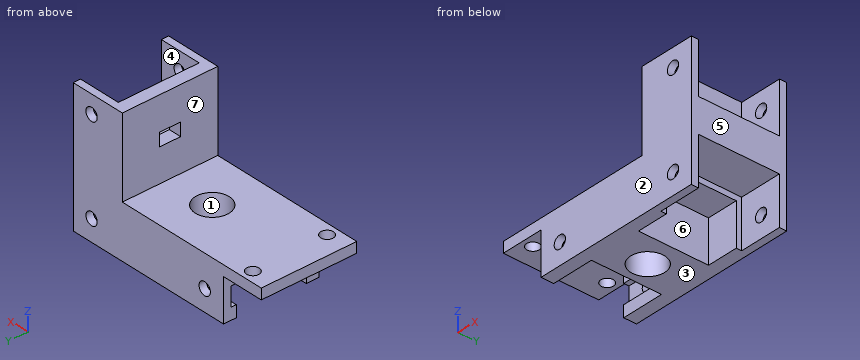
```python
from build123d import *

# Parameters (mm, degrees)
SKETCH1_W               = 36.85
SKETCH1_H               = 22.5
BOSS_EXTRUDE1_DEPTH     = 2.5
SKETCH2_W               = 21.3
SKETCH2_H               = 22.5
BOSS_EXTRUDE2_DEPTH     = 3
SKETCH3_W               = 21.3
SKETCH3_H               = 3
BOSS_EXTRUDE3_DEPTH     = 10
SKETCH4_W               = 49.85
SKETCH4_H               = 3
BOSS_EXTRUDE4_DEPTH     = 10
SKETCH8_W               = 3.1
SKETCH8_H               = 5
CUT_EXTRUDE1_DEPTH      = 5
SKETCH9_R               = 4
SKETCH9_R_2             = 1.5
CUT_EXTRUDE2_DEPTH      = 25
SKETCH11_W              = 10
SKETCH11_H              = 3
CUT_EXTRUDE3_DEPTH      = 10
SKETCH12_R              = 1.5
CUT_EXTRUDE4_DEPTH      = 10
SKETCH14_W              = 12.5
SKETCH14_H              = 10
SKETCH14_W_2            = 10
SKETCH14_H_2            = 8
BOSS_EXTRUDE8_DEPTH     = 19.5
SKETCH13_R              = 1.5
BOSS_EXTRUDE7_DEPTH     = 3
SKETCH15_R              = 4
CUT_EXTRUDE5_DEPTH      = 43
CUT_EXTRUDE6_DEPTH      = 17.7525
CUT_EXTRUDE6_DEPTH_BACK = 1.25
SKETCH16_W              = 10
SKETCH16_H              = 4.5
SKETCH17_W              = 14.131300264
SKETCH17_H              = 19.05
SKETCH17_W_2            = 13.234553728
CUT_EXTRUDE7_DEPTH      = 10


with BuildPart() as part:
    # Sketch1 → Boss-Extrude1 (new body)
    with BuildSketch(Plane.XY):
        with Locations((18.425, 11.25)):
            Rectangle(SKETCH1_W, SKETCH1_H)
    extrude(amount=BOSS_EXTRUDE1_DEPTH)

    # Sketch2 → Boss-Extrude2 (add)
    with BuildSketch(Plane(origin=(36.85, 0, 0), x_dir=(0, 0, -1), z_dir=(1, 0, 0))):
        with Locations((-10.65, 11.25)):
            Rectangle(SKETCH2_W, SKETCH2_H)
    extrude(amount=BOSS_EXTRUDE2_DEPTH)

    # Sketch3 → Boss-Extrude3 (add)
    with BuildSketch(Plane(origin=(39.85, 0, 0), x_dir=(0, 0, -1), z_dir=(1, 0, 0))):
        with Locations((-10.65, 1.5)):
            Rectangle(SKETCH3_W, SKETCH3_H)
    extrude(amount=BOSS_EXTRUDE3_DEPTH)

    # Sketch4 → Boss-Extrude4 (add)
    with BuildSketch(Plane(origin=(0, 0, 0), x_dir=(-1, 0, 0), z_dir=(0, 0, -1))):
        with Locations((-24.925, 1.5)):
            Rectangle(SKETCH4_W, SKETCH4_H)
    extrude(amount=BOSS_EXTRUDE4_DEPTH)

    # Sketch8 → Cut-Extrude1 (cut)
    with BuildSketch(Plane(origin=(39.85, 0, 0), x_dir=(0, 0, -1), z_dir=(1, 0, 0))):
        with Locations((-11.85, 11.25)):
            Rectangle(SKETCH8_W, SKETCH8_H)
    extrude(amount=-CUT_EXTRUDE1_DEPTH, mode=Mode.SUBTRACT)

    # Sketch9 → Cut-Extrude2 (cut)
    with BuildSketch(Plane.XY.offset(2.5)):
        with Locations((25.65, 11.25)):
            Circle(SKETCH9_R)
        with Locations((5.05, 20)):
            Circle(SKETCH9_R_2)
        with Locations((5.05, 2.5)):
            Circle(SKETCH9_R_2)
    extrude(amount=-CUT_EXTRUDE2_DEPTH, mode=Mode.SUBTRACT)

    # Sketch11 → Cut-Extrude3 (cut)
    with BuildSketch(Plane(origin=(0, 0, -10), x_dir=(-1, 0, 0), z_dir=(0, 0, -1))):
        with Locations((-5, 1.5)):
            Rectangle(SKETCH11_W, SKETCH11_H)
    extrude(amount=-CUT_EXTRUDE3_DEPTH, mode=Mode.SUBTRACT)

    # Sketch12 → Cut-Extrude4 (cut)
    with BuildSketch(Plane(origin=(0, 3, 0), x_dir=(1, 0, 0), z_dir=(0, 1, 0))):
        with Locations(Location((15, 5, 0), (0, 0, 270))):
            Circle(SKETCH12_R)
        with Locations(Location((45, 5, 0), (0, 0, 270))):
            Circle(SKETCH12_R)
        with Locations(Location((45, -17, 0), (0, 0, 270))):
            Circle(SKETCH12_R)
    extrude(amount=-CUT_EXTRUDE4_DEPTH, mode=Mode.SUBTRACT)

    # Sketch14 → Boss-Extrude8 (add)
    with BuildSketch(Plane(origin=(0, 3, 0), x_dir=(1, 0, 0), z_dir=(0, 1, 0))):
        with Locations((26.25, 5)):
            Rectangle(SKETCH14_W, SKETCH14_H)
        with Locations((44.85, -5.3)):
            Rectangle(SKETCH14_W_2, SKETCH14_H_2)
    extrude(amount=BOSS_EXTRUDE8_DEPTH)

    # Sketch13 → Boss-Extrude7 (add)
    with BuildSketch(Plane(origin=(0, 22.5, 0), x_dir=(1, 0, 0), z_dir=(0, 1, 0))):
        Polygon((10, 10), (49.85, 10), (49.85, 0), (49.85, -21.3), (39.85, -21.3), (39.85, 0), (10, 0), align=None)
        with Locations(Location((15, 5, 0), (0, 0, 270))):
            Circle(SKETCH13_R, mode=Mode.SUBTRACT)
        with Locations(Location((45, 5, 0), (0, 0, 270))):
            Circle(SKETCH13_R, mode=Mode.SUBTRACT)
        with Locations(Location((45, -17, 0), (0, 0, 270))):
            Circle(SKETCH13_R, mode=Mode.SUBTRACT)
    extrude(amount=-BOSS_EXTRUDE7_DEPTH)

    # Sketch15 → Cut-Extrude5 (cut)
    with BuildSketch(Plane.XY.offset(2.5)):
        with Locations((25.65, 11.25)):
            Circle(SKETCH15_R)
    extrude(amount=-CUT_EXTRUDE5_DEPTH, mode=Mode.SUBTRACT)

    # Sketch16 → Cut-Extrude6 (cut, two sides: drawn at the far end of the back side and taken through both)
    with BuildSketch(Plane.XZ.offset(-19.5).offset(-CUT_EXTRUDE6_DEPTH_BACK)):
        with Locations((15, -5)):
            Rectangle(SKETCH16_W, SKETCH16_H)
    extrude(amount=CUT_EXTRUDE6_DEPTH + CUT_EXTRUDE6_DEPTH_BACK, mode=Mode.SUBTRACT)

    # Sketch17 → Cut-Extrude7 (cut)
    with BuildSketch(Plane(origin=(49.85, 0, 0), x_dir=(0, 0, -1), z_dir=(1, 0, 0))):
        with Locations((-16.365650132, 11.25)):
            Rectangle(SKETCH17_W, SKETCH17_H)
        with Locations((5.317276864, 11.25)):
            Rectangle(SKETCH17_W_2, SKETCH17_H)
    extrude(amount=-CUT_EXTRUDE7_DEPTH, mode=Mode.SUBTRACT)


solid = part.part
```
Here's how the part is built. I have some questions about the finished solid (model axes, mm). Face numbers are marked on the shaded views. A direction names the side the tool comes from. Coordinates: 2 decimals unless noted, no trailing zeros. Order: outer loops, then holes, each group sorted by start corner. A loop starts at its lowest first (then second) coordinate and runs counter-clockwise, first axis right, second up. Notation, with made-up numbers: (89, -32.5) - (148, -32.5) arc R6 cw to (148, -28.5) - close; hole circle Ø7 at (-3, 79). An arc over 180 degrees is marked (long way). One line per question, with ' | ' between items.
(1) Suppose I cut it at B-B on y = 11.25. List the corners of the cut face in (x, z) for me.
Report:
outline: (0, 0) - (20, 0) - (20, -10) - (21.65, -10) - (21.65, 2.5) - (0, 2.5) - close; (29.65, -10) - (32.5, -10) - (32.5, 0) - (39.85, 0) - (39.85, 1.3) - (49.85, 1.3) - (49.85, 9.3) - (39.85, 9.3) - (39.85, 10.3) - (36.85, 10.3) - (36.85, 2.5) - (29.65, 2.5) - close; (36.85, 13.4) - (39.85, 13.4) - (39.85, 21.3) - (36.85, 21.3) - close
(2) Suppose I cut it at C-C on x = 5.05. List the corners of the cut face in (y, z) for me, and give its area (4 significant figures).
Report:
outline: (0, 0) - (1, 0) - (1, 2.5) - (0, 2.5) - close; (4, 0) - (18.5, 0) - (18.5, 2.5) - (4, 2.5) - close; (21.5, 0) - (22.5, 0) - (22.5, 2.5) - (21.5, 2.5) - close | area: 41.25 mm2
(3) Suppose I cut it at A-A on z = 17. List the corners of the cut face in (x, y) for me (3 decimals).
Report:
outline: (36.85, 0) - (43.5, 0) - (43.5, 1.725) - (39.85, 1.725) - (39.85, 20.775) - (43.5, 20.775) - (43.5, 22.5) - (36.85, 22.5) - close; (46.5, 0) - (49.85, 0) - (49.85, 1.725) - (46.5, 1.725) - close; (46.5, 20.775) - (49.85, 20.775) - (49.85, 22.5) - (46.5, 22.5) - close
(4) For the marked faces 4, 5, 6 and 7, which set-ups out of +Z, -Z, +X, -X, +Y, -Y let a thin tool reach every point of the face, with its end or its side?
Report:
face 4: +Z, +X | face 5: +Z, -Z, +X, +Y, -Y | face 6: -Z, +X | face 7: +Z, -X, +Y, -Y
(5) If we mould it in two halves opening along Y, with no side actions, what happens to the marked faces 1, 2 and 3? For each: pulls with the +Y half, pulls with the -Y half, needs draft (parallel to the pull), parting line crosses it, or undercut.
Report:
face 1: undercut | face 2: pulls with the -Y half | face 3: needs draft
(6) If I drill on L1, parallel to Y at x = 5.05, z = 1.8; L2, parallel to X at y = 21.45, z = -5; L3, parallel to Y at x = 25.65, z = -0.5, over which ranges is the centre line in solid material (lowest first)?
Report:
L1: y = 0 to 1, 4 to 18.5, 21.5 to 22.5 | L2: x = 10 to 13.5, 16.5 to 43.5, 46.5 to 49.85 | L3: y = 0 to 7.25, 15.25 to 22.5
(7) Will these pins go through, and if not, where does the flat tip stop? pin 1 (10 mm diameter, centred on y = 8, z = 13.5, fed in from -X); pin 2 (2 mm diameter, centred on x = 36, y = 8, fed in from -Z).
Report:
pin 1: stops at x = 36.85 | pin 2: stops at z = 0
(8) Suppose I cut it at D-D on z = -5. State how many separate pieces and enclosed holes the cut face has, and give its area (3 significant figures).
Report:
separate pieces: 5 | enclosed holes: 1 | area: 324 mm2
